from build123d import *

# Parameters (mm, degrees)
SKETCH2_W               = 25
SKETCH2_H               = 25
BOSS_EXTRUDE1_DEPTH     = 350
SKETCH3_R               = 1
CUT_EXTRUDE1_DEPTH      = 352.781181987
CUT_EXTRUDE2_DEPTH      = 352.781181987
CUT_EXTRUDE2_DEPTH_BACK = 352.781181987
SKETCH4_W               = 5
SKETCH4_H               = 25
SKETCH5_W               = 5
SKETCH5_H               = 25
CUT_EXTRUDE3_DEPTH      = 352.461235416


with BuildPart() as part:
    # Sketch2 → Boss-Extrude1 (new body)
    with BuildSketch(Plane(origin=(0, 0, 0), x_dir=(1, 0, 0), z_dir=(0, 1, 0))):
        with Locations((12.5, 12.5)):
            Rectangle(SKETCH2_W, SKETCH2_H)
    extrude(amount=BOSS_EXTRUDE1_DEPTH)

    # Sketch3 → Cut-Extrude1 (cut, through all)
    with BuildSketch(Plane.XY):
        with Locations((7.5, 342.5)):
            Circle(SKETCH3_R)
        with Locations((7.5, 297.5)):
            Circle(SKETCH3_R)
        with Locations((7.5, 277.5)):
            Circle(SKETCH3_R)
        with Locations((7.5, 257.5)):
            Circle(SKETCH3_R)
        with Locations(Location((17.5, 342.5, 0), (0, 0, 180))):
            Circle(SKETCH3_R)
        with Locations(Location((17.5, 297.5, 0), (0, 0, 180))):
            Circle(SKETCH3_R)
        with Locations(Location((17.5, 277.5, 0), (0, 0, 180))):
            Circle(SKETCH3_R)
        with Locations(Location((17.5, 257.5, 0), (0, 0, 180))):
            Circle(SKETCH3_R)
    extrude(amount=-CUT_EXTRUDE1_DEPTH, mode=Mode.SUBTRACT)

    # Sketch4 → Cut-Extrude2 (cut, two sides: drawn at the far end of the back side and taken through both)
    with BuildSketch(Plane.ZY.offset(-CUT_EXTRUDE2_DEPTH_BACK)):
        with Locations((-22.5, 12.5)):
            Rectangle(SKETCH4_W, SKETCH4_H)
        with Locations((-2.5, 12.5)):
            Rectangle(SKETCH4_W, SKETCH4_H)
    extrude(amount=CUT_EXTRUDE2_DEPTH + CUT_EXTRUDE2_DEPTH_BACK, mode=Mode.SUBTRACT)

    # Sketch5 → Cut-Extrude3 (cut, through all)
    with BuildSketch(Plane(origin=(0, 0, -20), x_dir=(-1, 0, 0), z_dir=(0, 0, -1))):
        with Locations((-22.5, 12.5)):
            Rectangle(SKETCH5_W, SKETCH5_H)
        with Locations((-2.5, 12.5)):
            Rectangle(SKETCH5_W, SKETCH5_H)
    extrude(amount=-CUT_EXTRUDE3_DEPTH, mode=Mode.SUBTRACT)


solid = part.part
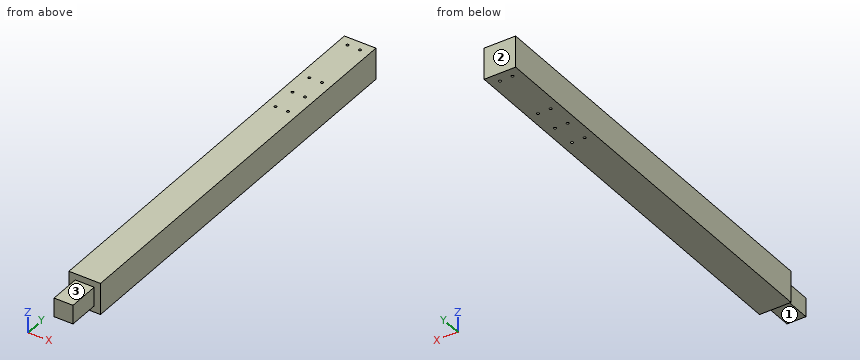
The model under review builds one solid part; all positions refer to its coordinate system, in mm. Face numbers are marked on the shaded views. A direction names the side the tool comes from. Give positions to 0.01 mm unless a question says otherwise; leave off trailing zeros. Put each result on its own line as item: value. Start each with the question number.
1. Wall thickness on probe 1 along X at (y, z) = (297.5, -19); probe 2 along Y at (x, z) = (7.5, -19.75); probe 3 along Y at (x, z) = (12.5, -2.5): over which ranges is each line inside the solid? List them lowest first.
2. For the marked faces 1, 2 and 3, list the 3-axis set-ups (+Z, -Z, +X, -X, +Y, -Y) from which the entire face can be reached by the end or side of a thin tool; tool diameter is ignored.
3. Clearance check with flat-ended pins moving along their axes: P1, Ø1.6, axis at x = 7.5, y = 257.5, coming from the +Z side; P2, Ø3, axis at x = 17.5, y = 297.5, coming from the -Z side; P3, Ø7.5, axis at x = 13, y = 14.5, coming from the +Z side. State where each tip first meets the part, or that it passes through.
4. We need section A-A on z = -8.25. State how many separate pieces and enclosed holes the cut face has, then the cut area to 3 significant figures.
Determined:
1. probe 1: 0 to 6.5, 8.5 to 16.5, 18.5 to 25
1. probe 2: 0 to 256.5, 258.5 to 276.5, 278.5 to 296.5, 298.5 to 341.5, 343.5 to 350
1. probe 3: 25 to 350
2. face 1: -Z, +X, -X, -Y
2. face 2: +Z, -Z, +X, -X, +Y
2. face 3: +Z, +X, -X, -Y
3. P1: through
3. P2: z = -25
3. P3: z = -5
4. separate pieces: 1
4. enclosed holes: 8
4. area: 8,470 mm^2
